Read the model definition and answer for the solid it produces. Units are mm, in the model's axes. Face numbers are marked on the shaded views. A direction names the side the tool comes from. Coordinates: 2 decimals unless noted, no trailing zeros. Loops run counter-clockwise (first coordinate to the right, second up) from the corner with the lowest first, then second, coordinate; pieces in that order, holes last. Notation, with made-up numbers: (89, 28) -> (114, 28) arc R10 ccw to (114, 39) -> close; hole circle Ø10 at (-33, 55). An arc over 180 degrees is marked (long way). Answer as CSV lines item,"result".
```python
from build123d import *

# Parameters (mm, degrees)
CYLINDER007_R          = 3
CYLINDER007_DEPTH      = 10
CYLINDER004_R          = 2.1
CYLINDER004_DEPTH      = 10
CYLINDER003_R          = 2.1
CYLINDER003_DEPTH      = 10
BOX001_W               = 7
BOX001_H               = 8
BOX001_DEPTH           = 17
BOX001_PLACEMENT_ANGLE = 9
SKETCH002_R            = 6.5
SKETCH002_R_2          = 1.98925
PAD002_DEPTH           = 4
CYLINDER006_R          = 2.1
CYLINDER006_DEPTH      = 10
CYLINDER005_R          = 2.1
CYLINDER005_DEPTH      = 10
BOX002_W               = 7
BOX002_H               = 8
BOX002_DEPTH           = 17
BOX002_PLACEMENT_ANGLE = 9
CUT003_PLACEMENT_ANGLE = 180


with BuildPart() as cylinder007:
    # Cylinder007 → Cylinder007 (new body)
    with BuildSketch(Plane(origin=(9, -52.5, 44), x_dir=(0, 0, -1), z_dir=(1, 0, 0))):
        Circle(CYLINDER007_R)
    extrude(amount=CYLINDER007_DEPTH)


with BuildPart() as cylinder004:
    # Cylinder004 → Cylinder004 (new body)
    with BuildSketch(Plane(origin=(23, 39.6, 42.2), x_dir=(0, 0, -1), z_dir=(1, 0, 0))):
        Circle(CYLINDER004_R)
    extrude(amount=CYLINDER004_DEPTH)


with BuildPart() as fusion001:
    # Cylinder003 → Cylinder003 (new body)
    with BuildSketch(Plane(origin=(23, 38, 32.3), x_dir=(0, 0, -1), z_dir=(1, 0, 0))):
        Circle(CYLINDER003_R)
    extrude(amount=CYLINDER003_DEPTH)

    # Fusion001: union Cylinder004
    add(cylinder004.part)


with BuildPart() as fusion001_1:
    # Fusion001 placement: moved
    add(fusion001.part.moved(Location((-1, 0, 0))))


with BuildPart() as cut002:
    # Box001 → Box001 (new body)
    with BuildSketch(Plane.XY):
        with Locations((3.5, 4)):
            Rectangle(BOX001_W, BOX001_H)
    extrude(amount=BOX001_DEPTH)


with BuildPart() as cut002_1:
    # Box001 placement: moved
    add(cut002.part.moved(Location((20.2, 33, 29.5))).rotate(Axis((20.2, 33, 29.5), (-1, 0, 0)), BOX001_PLACEMENT_ANGLE))

    # Cut002: cut Fusion001
    add(fusion001_1.part, mode=Mode.SUBTRACT)


with BuildPart() as obj1:
    # Sketch002 → Pad002 (new body)
    with BuildSketch(Plane.YZ):
        with BuildLine():
            Line((-19.485119, 0), (59.609761, 0))
            ThreePointArc((59.609761, 0), (71.609761, 12), (59.609761, 24))
            Line((-19.485119, 36), (59.609761, 24))
            ThreePointArc((-19.485119, 36), (-37.485119, 18), (-19.485119, 0))
        make_face()
        with Locations((50, 13.528694)):
            Circle(SKETCH002_R, mode=Mode.SUBTRACT)
        with Locations((-27.485119, 18)):
            Circle(SKETCH002_R_2, mode=Mode.SUBTRACT)
    extrude(amount=PAD002_DEPTH)


with BuildPart() as obj1_1:
    # Body002 placement: moved
    add(obj1.part.moved(Location((18, -25, 26))))


with BuildPart() as cylinder006:
    # Cylinder006 → Cylinder006 (new body)
    with BuildSketch(Plane(origin=(23, 39.6, 42.2), x_dir=(0, 0, -1), z_dir=(1, 0, 0))):
        Circle(CYLINDER006_R)
    extrude(amount=CYLINDER006_DEPTH)


with BuildPart() as fusion002:
    # Cylinder005 → Cylinder005 (new body)
    with BuildSketch(Plane(origin=(23, 38, 32.3), x_dir=(0, 0, -1), z_dir=(1, 0, 0))):
        Circle(CYLINDER005_R)
    extrude(amount=CYLINDER005_DEPTH)

    # Fusion002: union Cylinder006
    add(cylinder006.part)


with BuildPart() as fusion002_1:
    # Fusion002 placement: moved
    add(fusion002.part.moved(Location((-1, 0, 0))))


with BuildPart() as cut004:
    # Box002 → Box002 (new body)
    with BuildSketch(Plane.XY):
        with Locations((3.5, 4)):
            Rectangle(BOX002_W, BOX002_H)
    extrude(amount=BOX002_DEPTH)


with BuildPart() as cut004_1:
    # Box002 placement: moved
    add(cut004.part.moved(Location((20.2, 33, 29.5))).rotate(Axis((20.2, 33, 29.5), (-1, 0, 0)), BOX002_PLACEMENT_ANGLE))

    # Cut003: cut Fusion002
    add(fusion002_1.part, mode=Mode.SUBTRACT)


with BuildPart() as cut004_2:
    # Cut003 placement: moved
    add(cut004_1.part.moved(Location((0, 29.8756, 81.7462))).rotate(Axis((0, 29.8756, 81.7462), (1, 0, 0)), CUT003_PLACEMENT_ANGLE))

    # Fusion003: union Cut002, obj1
    add(cut002_1.part)
    add(obj1_1.part)

    # Cut004: cut Cylinder007
    add(cylinder007.part, mode=Mode.SUBTRACT)


solid = cut004_2.part
```
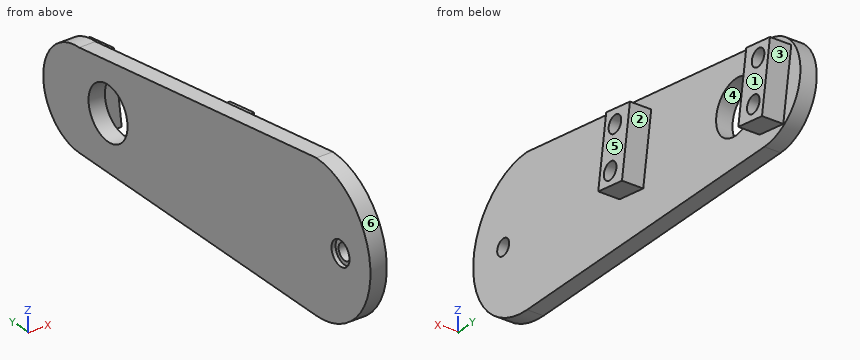
Q1. A cutting plane is placed at C-C, the plane y = -52.5. Write down the section's boundary in (x, z), and give its area (3 significant figures).
Results:
outline,"(18, 27.88) -> (22, 27.88) -> (22, 42.01) -> (19, 42.01) -> (19, 41) -> (18, 41) -> close; (18, 47) -> (19, 47) -> (19, 45.99) -> (22, 45.99) -> (22, 60.12) -> (18, 60.12) -> close"
area,"111 mm²"
Q2. A cutting plane is placed at A-A, the plane x = 25. Write down the section's boundary in (y, z).
Results:
outline,"(-13.69, 36.71) -> (-5.78, 35.46) -> (-3.12, 52.25) -> (-11.03, 53.5) -> close; (33, 29.5) -> (40.9, 28.25) -> (43.56, 45.04) -> (35.66, 46.29) -> close; hole circle Ø4.2 at (-9.72, 39.55); hole circle Ø4.2 at (-8.12, 49.45); hole circle Ø4.2 at (38, 32.3); hole circle Ø4.2 at (39.6, 42.2)"
Q3. Given pin 1 Ø18 at (y, z) = (13, 42) entering from +X; pin 2 Ø1 at (x, z) = (20.5, 30.5) entering from -Y (3 decimals); pin 3 Ø1.5 at (x, y) = (24, -8) entering from -Z, each flat-ended and moving along its own axis, determine where each tip first touches the part or whether it passes through.
Results:
pin 1,"stops at x = 22"
pin 2,"stops at y = -56.935"
pin 3,"stops at z = 35.69"
Q4. For the marked faces 1, 2 and 3, determine the directions among +Z, -Z, +X, -X, +Y, -Y from which every point of the face is accessible in a straight line to the end or side of a thin tool.
Results:
face 1,"+Z, -Z, +X, +Y, -Y"
face 2,"-Z, +X"
face 3,"-Z, +X, +Y"
Q5. A cutting plane is placed at B-B, the plane y = 23. Write down the section's boundary in (x, z), and give its area (3 significant figures).
Results:
outline,"(18, 26) -> (22, 26) -> (22, 33.34) -> (18, 33.34) -> close; (18, 45.71) -> (22, 45.71) -> (22, 51.76) -> (18, 51.76) -> close"
area,"53.6 mm²"
Q6. A cutting plane is placed at D-D, the plane x = 20.25. Write down the section's boundary in (y, z).
Results:
outline,"(-44.49, 26) -> (34.61, 26) arc R12 ccw to (34.61, 50) -> (-44.49, 62) arc R18 ccw to start; hole circle Ø3.98 at (-52.49, 44); hole circle Ø13 at (25, 39.53)"
Q7. For a pull along Z with two mould halves and no side action, classify the marked faces 4, 5 and 6 as pulls with the +Z half, pulls with the -Z half, needs draft (parallel to the pull), parting line crosses it, or undercut.
Results:
face 4,"undercut"
face 5,"needs draft"
face 6,"parting line crosses it"
Q8. Find the intervals of material crossed by probe 1 along Z at (x, y) = (23.6, 38); probe 2 along Y at (x, z) = (26.1, 42.2); probe 3 along Z at (x, y) = (24.8, 39.6), in increasing order. Write a range as [from, to].
Results:
probe 1,"z = [28.71, 30.2], [34.4, 40.84], [43.56, 45.92]"
probe 2,"y = [-12.82, -4.72], [35.01, 37.5], [41.7, 43.11]"
probe 3,"z = [28.45, 30.94], [33.66, 40.1], [44.3, 45.67]"
